Can you work these out from the drawing? Everything is in mm from the part's minimum corner. Coordinates: 2 decimals unless noted, no trailing zeros. Order: outer loops, then holes, each group sorted by start corner. A loop starts at its lowest first (then second) coordinate and runs counter-clockwise, first axis right, second up. Notation, with made-up numbers: (17.5, 72.25) -> (67.5, 72.25) arc R19 ccw to (67.5, 85.25) -> close; hole circle Ø4 at (12, -29.75). An arc over 180 degrees is marked (long way). Put each result on its own line as item: value. Start each with the question number.
Q1. We'd pull the mould along Z, two halves only. Please class the marked faces 1, 2 and 3: +Z half, -Z half, draft (parallel to the pull), parting line (faces both ways), or undercut.
Q2. If we section it at A-A (z = 22.5): Please give me the cut outline in (x, y).
Q3. If we section it at C-C (y = 4.5): Count the separate pieces of the cut face and the enclosed holes in it, and give its area (3 significant figures).
Q4. Will these pins go through, and if not, where does the flat tip stop? pin 1 (6 mm diameter, centred on y = 3, z = 21.5, fed in from +X); pin 2 (12 mm diameter, centred on x = 13, y = 9.5, fed in from -Z); pin 3 (2 mm diameter, centred on x = 14, y = 4, fed in from +Z).
Q5. Please list where these lines run through material, in increasing order: line 1 along X through (y, z) = (11, 22.5); line 2 along Z through (x, y) = (31.5, 5.5) (1 decimal); line 3 along X through (y, z) = (16.25, 7.5).
Q6. If we section it at B-B (x = 22.5): Please give me the cut outline in (y, z).
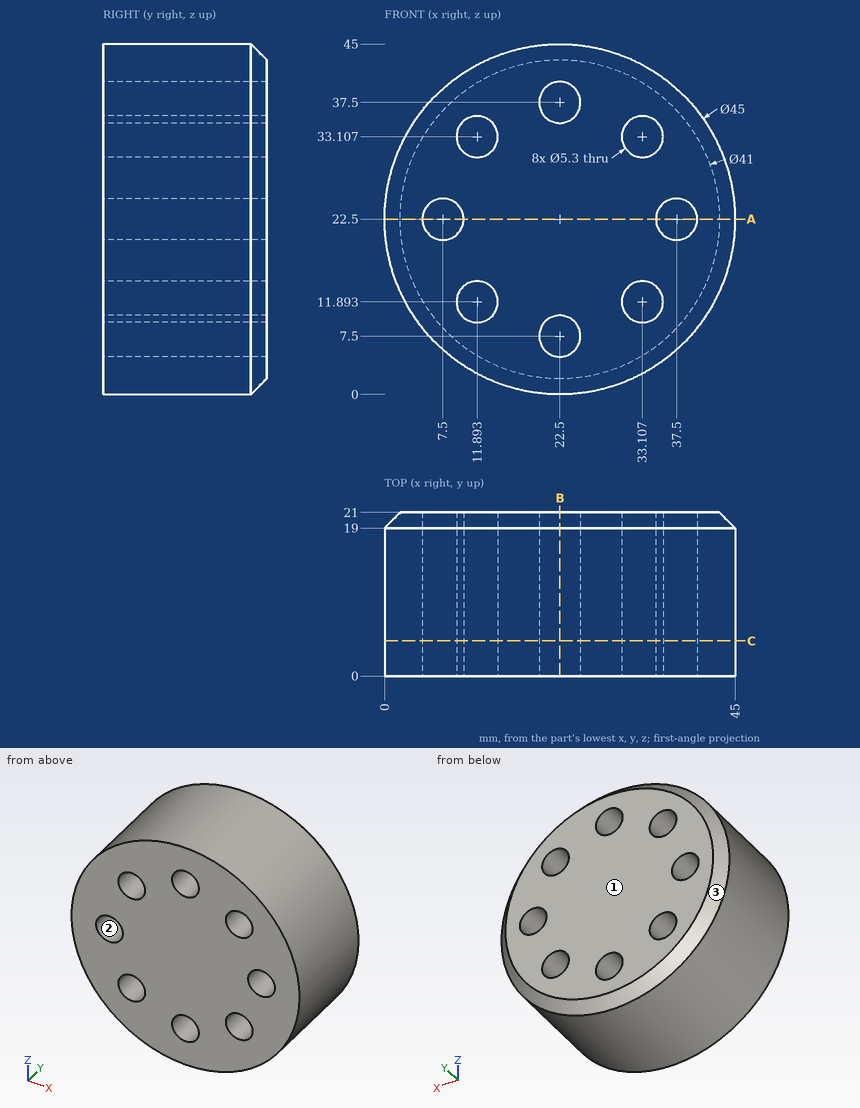
The answers:
1. face 1: draft
1. face 2: undercut
1. face 3: parting line
2. outline: (0, 0) -> (4.85, 0) -> (4.85, 21) -> (2, 21) -> (0, 19) -> close; (10.15, 0) -> (34.85, 0) -> (34.85, 21) -> (10.15, 21) -> close; (40.15, 0) -> (45, 0) -> (45, 19) -> (43, 21) -> (40.15, 21) -> close
3. separate pieces: 1
3. enclosed holes: 8
3. area: 1,410 mm^2
4. pin 1: x = 45
4. pin 2: z = 0.27
4. pin 3: z = 43.71
5. line 1: 0 to 4.85, 10.15 to 34.85, 40.15 to 45
5. line 2: 1.9 to 9.8, 14 to 31, 35.2 to 43.1
5. line 3: 5.73 to 19.85, 25.15 to 39.27
6. outline: (0, 0) -> (19, 0) -> (21, 2) -> (21, 4.85) -> (0, 4.85) -> close; (0, 10.15) -> (21, 10.15) -> (21, 34.85) -> (0, 34.85) -> close; (0, 40.15) -> (21, 40.15) -> (21, 43) -> (19, 45) -> (0, 45) -> close
